Geometry: see drawing. Coordinates: mm, zero at the bounding-box minimum. A direction names the side the tool comes from. Round coordinates to 2 decimals unless told otherwise and drop trailing zeros. Order: outer loops, then holes, each group sorted by start corner. A loop starts at its lowest first (then second) coordinate and runs counter-clockwise, first axis right, second up.
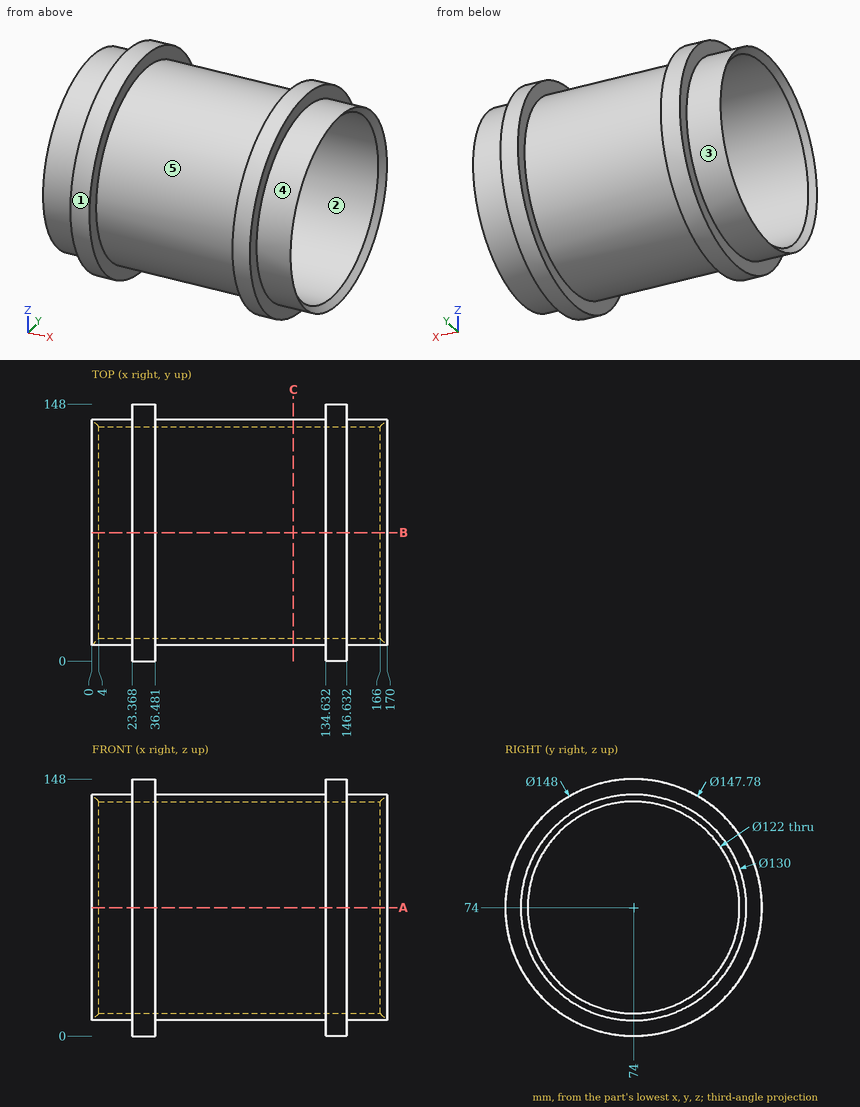
1. Access query for the marked faces 3, 4 and 5. Directions: +Z, -Z, +X, -X, +Y, -Y. A direction counts if a zero-diameter tool reaches every point of the face in a straight line with its end or side. Return the directions, or none.
2. Pull-direction query (Z, two-part tool) for the marked faces 1 and 2; classes: released by +Z, released by -Z, zero draft, split by the parting line, or undercut.
3. First-contact query: pin 1 (4 mm diameter, centred on x = 112, y = 72, fed in from -Z); pin 2 (12 mm diameter, centred on x = 20.5, y = 36, fed in from -Z); pin 3 (1 mm diameter, centred on x = 102.5, y = 61.5, fed in from -Z). Flat tips, straight axial feed; report the tip coordinate or a pass-through.
4. Section C-C on x = 116. Return loops of the section in (y, z).
5. Line query: line 1 along Z through (x, y) = (51, 74); line 2 along X through (y, z) = (102.5, 140); line 3 along Y through (x, z) = (114.5, 29) (1 decimal). Output: solid intervals per line, ascending.
6. Section A-A on z = 74. Return loops of the section in (x, y), plus the area to 3 significant figures.
Result:
1. face 3: -X
1. face 4: +X
1. face 5: none
2. face 1: split by the parting line
2. face 2: undercut
3. pin 1: stops at z = 9
3. pin 2: stops at z = 7.63
3. pin 3: stops at z = 10.12
4. outline: circle Ø130 at (74, 74); hole circle Ø122 at (74, 74)
5. line 1: z = 9 to 13, 135 to 139
5. line 2: x = 23.37 to 36.48, 134.63 to 146.63
5. line 3: y = 27.1 to 32.8, 115.2 to 120.9
6. outline: (0, 9) - (23.37, 9) - (23.37, 0) - (36.48, 0) - (36.48, 9) - (134.63, 9) - (134.63, 0.11) - (146.63, 0.11) - (146.63, 9) - (170, 9) - (166, 13) - (4, 13) - close; (0, 139) - (4, 135) - (166, 135) - (170, 139) - (146.63, 139) - (146.63, 147.89) - (134.63, 147.89) - (134.63, 139) - (36.48, 139) - (36.48, 148) - (23.37, 148) - (23.37, 139) - close
6. area: 1,780 mm2
